Read the model definition and answer for the solid it produces. Units are mm, in the model's axes. A direction names the side the tool comes from. Round coordinates to 2 decimals unless told otherwise and drop trailing zeros. Order: outer loops, then holes, each group sorted by start corner. A loop starts at its lowest first (then second) coordinate and runs counter-clockwise, first axis right, second up. Notation, with made-up numbers: (43.5, 57) - (51.5, 57) arc R14 cw to (51.5, 63) - close; hole circle Ø2 at (3.25, 2.5). An arc over 180 degrees is marked (long way). Put each result on its own line as item: value. Start each with the question number.
Q1. Find the intervals of material crossed by line 1 along X through (y, z) = (18, 4); line 2 along Z through (x, y) = (-5, 72.5); line 3 along Z through (x, y) = (-12.5, 189.5), in increasing order. Write a range as from..to.
Q2. Each of these flat-tipped pins is pushed along its axis until it touches: pin 1 Ø12 at (x, z) = (-14.5, 12.5) entering from -Y; pin 2 Ø1.5 at (x, y) = (-16, 158.5) entering from -Z; pin 3 Ø3.5 at (x, y) = (-2.5, 54.5) entering from -Z; pin 4 Ø6 at (x, z) = (-16.5, 8) entering from +Y. Where does it stop, or does it pass through?
Q3. Which of the six approach directions +Z, -Z, +X, -X, +Y, -Y give full straight-line access (tool end or side, diameter ignored) to faces 4 (the face through (20.5, 99, 7)), 5 (the face through (-21.5, 99, 11))?
Q4. Section D-D on y = 95 is taken. State how many separate pieces and enclosed holes the cut face has, then the cut area to 3 significant figures.
Q5. Section B-B on z = 10.75 is taken. Give the vertices of the cut face in (x, y).
Q6. Section A-A on x = 16 is taken. Give the vertices of the cut face in (y, z), then the cut area to 3 significant figures.
Q7. For a pull along Z with two mould halves and no side action, classify faces 1 (the face through (7, 99, 0)), 2 (the face through (-14, 99, 21)), 3 (the face through (12, 99, 22)) as pulls with the +Z half, pulls with the -Z half, needs draft (parallel to the pull), parting line crosses it, or undercut.
Q8. Section C-C on x = -0.5 is taken. Give the vertices of the cut face in (y, z).
from build123d import *

# Parameters (mm, degrees)
F1_DEPTH = 200


# Not quite as in the source:
# - a pattern or mirror of a feature is missing from the dataset's text; its kind, count and spacing are read off the source's solid


with BuildPart() as f1:
    # F0 (on Front) → F1 (new body)
    with BuildSketch(Plane.XZ):
        with BuildLine():
            ThreePointArc((-3.9, 21.5), (-4.0464466094, 21.8535533906), (-4.4, 22))
            Line((-4.4, 22), (-20, 22))
            ThreePointArc((-20, 22), (-21.0606601718, 21.5606601718), (-21.5, 20.5))
            Line((-21.5, 20.5), (-21.5, 1.5))
            ThreePointArc((-21.5, 1.5), (-21.0606601718, 0.4393398282), (-20, 0))
            Line((-20, 0), (-18.4, 0))
            ThreePointArc((-18.4, 0), (-18.0464466094, 0.1464466094), (-17.9, 0.5))
            ThreePointArc((-17.9, 0.5), (-18.0464466094, 0.8535533906), (-18.4, 1))
            Line((-18.4, 1), (-20, 1))
            ThreePointArc((-20, 1), (-20.3535533906, 1.1464466094), (-20.5, 1.5))
            Line((-20.5, 1.5), (-20.5, 12.4))
            ThreePointArc((-20.5, 12.4), (-20.3535533906, 12.7535533906), (-20, 12.9))
            Line((-20, 12.9), (-8, 12.9))
            ThreePointArc((-8, 12.9), (-7.6464466094, 12.7535533906), (-7.5, 12.4))
            Line((-7.5, 12.4), (-7.5, 1.5))
            ThreePointArc((-7.5, 1.5), (-7.6464466094, 1.1464466094), (-8, 1))
            Line((-8, 1), (-9.6, 1))
            ThreePointArc((-9.6, 1), (-9.9535533906, 0.8535533906), (-10.1, 0.5))
            ThreePointArc((-10.1, 0.5), (-9.9535533906, 0.1464466094), (-9.6, 0))
            Line((-9.6, 0), (-4.4, 0))
            ThreePointArc((-4.4, 0), (-4.0464466094, 0.1464466094), (-3.9, 0.5))
            ThreePointArc((-3.9, 0.5), (-4.0464466094, 0.8535533906), (-4.4, 1))
            Line((-4.4, 1), (-6, 1))
            ThreePointArc((-6, 1), (-6.3535533906, 1.1464466094), (-6.5, 1.5))
            Line((-6.5, 1.5), (-6.5, 12.4))
            ThreePointArc((-6.5, 12.4), (-6.3535533906, 12.7535533906), (-6, 12.9))
            Line((-6, 12.9), (0, 12.9))
            Line((0, 12.9), (0, 13.9))
            Line((0, 13.9), (-6, 13.9))
            ThreePointArc((-6, 13.9), (-6.3535533906, 14.0464466094), (-6.5, 14.4))
            Line((-6.5, 14.4), (-6.5, 20.5))
            ThreePointArc((-6.5, 20.5), (-6.3535533906, 20.8535533906), (-6, 21))
            Line((-6, 21), (-4.4, 21))
            ThreePointArc((-4.4, 21), (-4.0464466094, 21.1464466094), (-3.9, 21.5))
        make_face()
        with BuildLine():
            Line((-8, 13.9), (-20, 13.9))
            ThreePointArc((-20, 13.9), (-20.3535533906, 14.0464466094), (-20.5, 14.4))
            Line((-20.5, 14.4), (-20.5, 20.5))
            ThreePointArc((-20.5, 20.5), (-20.3535533906, 20.8535533906), (-20, 21))
            Line((-20, 21), (-8, 21))
            ThreePointArc((-8, 21), (-7.6464466094, 20.8535533906), (-7.5, 20.5))
            Line((-7.5, 20.5), (-7.5, 14.4))
            ThreePointArc((-7.5, 14.4), (-7.6464466094, 14.0464466094), (-8, 13.9))
        make_face(mode=Mode.SUBTRACT)
    extrude(amount=-F1_DEPTH)

    # F1_copies: F1 across plane


with BuildPart() as f1_1:
    add(f1.part)
    add(f1.part.mirror(Plane(origin=(0, 0, 0), x_dir=(0, 0, 1), z_dir=(1, 0, 0))))


solid = f1_1.part
Findings:
1. line 1: -21.5..-20.5, -7.5..-6.5, 6.5..7.5, 20.5..21.5
1. line 2: 0..1, 12.9..13.9, 21..22
1. line 3: 12.9..13.9, 21..22
2. pin 1: y = 0
2. pin 2: z = 12.9
2. pin 3: z = 0.02
2. pin 4: through
3. face 4: +Y, -Y
3. face 5: +Z, -Z, -X, +Y, -Y
4. separate pieces: 1
4. enclosed holes: 2
4. area: 172 mm2
5. outline: (-21.5, 0) - (-20.5, 0) - (-20.5, 200) - (-21.5, 200) - close; (-7.5, 0) - (-6.5, 0) - (-6.5, 200) - (-7.5, 200) - close; (6.5, 0) - (7.5, 0) - (7.5, 200) - (6.5, 200) - close; (20.5, 0) - (21.5, 0) - (21.5, 200) - (20.5, 200) - close
6. outline: (0, 12.9) - (200, 12.9) - (200, 13.9) - (0, 13.9) - close; (0, 21) - (200, 21) - (200, 22) - (0, 22) - close
6. area: 400 mm2
7. face 1: pulls with the -Z half
7. face 2: undercut
7. face 3: pulls with the +Z half
8. outline: (0, 12.9) - (200, 12.9) - (200, 13.9) - (0, 13.9) - close
